Autodesk Inventor part; units mm, degrees
ref_plane "YZ Plane" through (0, 0, 0) normal (1, 0, 0) x (0, 1, 0)
ref_plane "XZ Plane" through (0, 0, 0) normal (0, 1, 0) x (-1, 0, 0)
ref_plane "XY Plane" through (0, 0, 0) normal (0, 0, 1) x (1, 0, 0)
sketch "Sketch1" plane through (0, 0, 0) normal (0, 0, 1) x (1, 0, 0)
  circle A0 centre (0, 0) radius 0.95
  circle A1 centre (0, 0) radius 1.95
  dimension "d0" = 1.9
  dimension "d1" = 3.9
extrude "Extrusion1" add sketch "Sketch1" along normal blind 6.3
sketch "Sketch2" plane through (0, 0, 6.3) normal (0, 0, 1) x (1, 0, 0)
  line L0 (-2.75, -2.75) -> (2.75, -2.75)
  line L1 (2.75, -2.75) -> (2.75, 2.75)
  line L2 (2.75, 2.75) -> (-2.75, 2.75)
  line L3 (-2.75, 2.75) -> (-2.75, -2.75)
  line L4 (-2.75, -2.75) -> (2.75, 2.75) construction
  line L5 (2.75, -2.75) -> (-2.75, 2.75) construction
  point P0 (0, 0)
  dimension "d4" = 5.5
  dimension "d5" = 5.5
extrude "Extrusion2" add sketch "Sketch2" along normal blind 3.7
extrude "Extrusion3" cut sketch "Sketch1" along normal through all contours A0
sketch "Sketch3" plane through (-2.75, 2.75, 6.3) normal (0, 1, 0) x (1, 0, 0)
  line L0 (0.8, 6.3) -> (0.8, 0)
  line L1 (0, 0) -> (0, -3.7)
  line L2 (0, -3.7) -> (5.5, -3.7)
  line L3 (0, -3.7) -> (0.8, -3.7)
  line L4 (6.7827, -4.1433) -> (6.7693, -4.1433)
  line L5 (0.8, -3.7) -> (0.8, -21.7)
  line L6 (0.8, -21.7) -> (0, -21.7)
  line L7 (0, -21.7) -> (0, -3.7)
  line L8 (2.75, -3.7) -> (2.75, -2.5481)
  line L9 (4.7, -3.7) -> (4.7, -21.7)
  line L10 (4.7, -21.7) -> (5.5, -21.7)
  line L11 (5.5, -21.7) -> (5.5, -3.7)
  point P0 (2.75, 6.3)
  dimension "d10" = 18
extrude "Extrusion4" add sketch "Sketch3" against normal up to surface (5.5 mm away)
sketch "Sketch4" plane through (-2.75, -2.75, 6.3) normal (-1, 0, 0) x (0, 0, 1)
  line L0 (21.7, 5.5) -> (21.7, 0)
  line L1 (21.7, 2.75) -> (19.1, 2.75)
  circle A0 centre (16.5832, 2.75) radius 0.86
  point P0 (-6.3, 2.75)
  dimension "d13" = 2.6
  dimension "d14" = 1.72
extrude "Extrusion5" add sketch "Sketch4" against normal up to surface (5.5 mm away)
fillet "Fillet1" radius 2.6 2 edges at (-2.35, -2.75, 28) (-2.35, 2.75, 28)
fillet "Fillet2" radius 2.6 2 edges at (2.35, 2.75, 28) (2.35, -2.75, 28)
properties part number "G"
Input: part model. Units: mm. Frame: model coordinates. A direction names the side the tool comes from. Round coordinates to 2 decimals unless told otherwise and drop trailing zeros. Order: outer loops, then holes, each group sorted by start corner. A loop starts at its lowest first (then second) coordinate and runs counter-clockwise, first axis right, second up. Notation, with made-up numbers: (28.25, 56) - (67.25, 56) arc R30 ccw to (67.25, 89) - close; hole circle Ø10 at (-16, 52). An arc over 180 degrees is marked (long way). Use a Markdown table: item, result.
1. Section B-B on z = 26. Return the cut outline in (x, y).
Evaluation:
| item | result |
|---|---|
| outline | (-2.75, -2.68) - (-1.95, -2.68) - (-1.95, 2.68) - (-2.75, 2.68) - close; (1.95, -2.68) - (2.75, -2.68) - (2.75, 2.68) - (1.95, 2.68) - close |
2. Access query for faces 4 (the face through (-0.027, 0.258, 23.703)), 5 (the face through (-0.95, -0.04, 4.93)), 6 (the face through (-2.75, 0, 17)), 7 (the face through (-1, 1, 10)). Directions: +Z, -Z, +X, -X, +Y, -Y. A direction counts if a zero-diameter tool reaches every point of the face in a straight line with its end or side. Return the directions, or none.
Evaluation:
| item | result |
|---|---|
| face 4 | none |
| face 5 | -Z |
| face 6 | +Z, -Z, -X, +Y, -Y |
| face 7 | +Y, -Y |
3. Section A-A on x = 0. Return the cut outline in (y, z), then the cut area to 3 significant figures.
Evaluation:
| item | result |
|---|---|
| outline | (-2.75, 6.3) - (-1.95, 6.3) - (-1.95, 0) - (-0.95, 0) - (-0.95, 10) - (-2.75, 10) - close; circle Ø1.72 at (0, 22.88); (0.95, 0) - (1.95, 0) - (1.95, 6.3) - (2.75, 6.3) - (2.75, 10) - (0.95, 10) - close |
| area | 28.2 mm^2 |
4. First-contact query: pin 1 (1.7 mm diameter, centred on x = 0, y = 0, fed in from -Z); pin 2 (1.2 mm diameter, centred on x = 0, y = 0, fed in from +Z); pin 3 (1.5 mm diameter, centred on x = -1, y = -2, fed in from +Z). Flat tips, straight axial feed; report the tip coordinate or a pass-through.
Evaluation:
| item | result |
|---|---|
| pin 1 | z = 22.02 |
| pin 2 | z = 23.74 |
| pin 3 | z = 10 |
5. Section C-C on x = -1.55. Return the cut outline in (y, z).
Evaluation:
| item | result |
|---|---|
| outline | (-2.75, 6.3) - (-1.18, 6.3) - (-1.18, 0) - (1.18, 0) - (1.18, 6.3) - (2.75, 6.3) - (2.75, 10) - (-2.75, 10) - close; circle Ø1.72 at (0, 22.88) |
6. Section D-D on y = 0.5. Return the cut outline in (x, z).
Evaluation:
| item | result |
|---|---|
| outline | (-2.75, 6.3) - (-1.88, 6.3) - (-1.88, 0) - (-0.81, 0) - (-0.81, 10) - (-1.95, 10) - (-1.95, 22.18) - (1.95, 22.18) - (1.95, 10) - (0.81, 10) - (0.81, 0) - (1.88, 0) - (1.88, 6.3) - (2.75, 6.3) - (2.75, 27.98) - (1.95, 27.98) - (1.95, 23.58) - (-1.95, 23.58) - (-1.95, 27.98) - (-2.75, 27.98) - close |
7. Mould query, pull axis Z, two halves, no side actions, for faces 1 (the face through (-2.5, -2.75, 11.5)), 2 (the face through (-1.95, 0, 19)), 3 (the face through (-2.356, -2.009, 27.218)). Classes: +Z half, -Z half, draft (parallel to the pull), parting line (faces both ways), or undercut.
Evaluation:
| item | result |
|---|---|
| face 1 | draft |
| face 2 | undercut |
| face 3 | +Z half |
8. Material intervals for probe 1 along X at (y, z) = (0.4, 25.5); probe 2 along Y at (x, z) = (-0.1, 9.75); probe 3 along Z at (x, y) = (-2.05, -0.1), sorted ascending.
Evaluation:
| item | result |
|---|---|
| probe 1 | -2.75 to -1.95, 1.95 to 2.75 |
| probe 2 | -2.75 to -0.94, 0.94 to 2.75 |
| probe 3 | 6.3 to 28 |
